Autodesk Inventor part; units mm, degrees
ref_plane "YZ Plane" through (0, 0, 0) normal (1, 0, 0) x (0, 1, 0)
ref_plane "XZ Plane" through (0, 0, 0) normal (0, 1, 0) x (-1, 0, 0)
ref_plane "XY Plane" through (0, 0, 0) normal (0, 0, 1) x (1, 0, 0)
sketch "Sketch1" plane through (0, 0, 0) normal (0, 0, 1) x (1, 0, 0)
  line L0 (0, 0) -> (13, 0)
  line L1 (13, 0) -> (13, 80)
  line L2 (13, 80) -> (0, 80)
  line L3 (0, 80) -> (0, 0)
  dimension "d0" = 80
  dimension "d1" = 13
extrude "Extrusion1" add sketch "Sketch1" along normal blind 58
sketch "Sketch2" plane through (0, 0, 58) normal (0, 0, 1) x (1, 0, 0)
  line L0 (10, 77) -> (3, 77)
  line L1 (3, 3) -> (10, 3)
  line L2 (10, 3) -> (10, 77)
  line L3 (13, 0) -> (13, 80)
  line L4 (13, 80) -> (0, 80)
  line L5 (0, 0) -> (13, 0)
  line L6 (0, 80) -> (0, 0)
  line L7 (0, 10) -> (3, 10)
  line L8 (3, 70) -> (0, 70)
  line L9 (0, 70) -> (0, 10)
  line L10 (3, 77) -> (3, 70)
  line L11 (3, 10) -> (3, 3)
  point P0 (0, 70)
  dimension "d4" = 3
  dimension "d5" = 3
  dimension "d6" = 3
  dimension "d8" = 10
  dimension "d9" = 10
extrude "Extrusion2" cut sketch "Sketch2" against normal through all contours L2 L1 L11 L7 L6 L8 L10 L0
sketch "Sketch3" plane through (13, 0, 0) normal (1, 0, 0) x (0, 0, -1)
  circle A0 centre (-40, 40) radius 4
  line L0 (-58, 0) -> (-58, 80)
  line L1 (0, 0) -> (-58, 0)
  line L2 (0, 0) -> (0, 80)
  dimension "d12" = 8
  dimension "d14" = 40
  dimension "d17" = 40
extrude "Extrusion3" cut sketch "Sketch3" against normal through all
properties part number "servo_mount" material "PC/ABS Plastic"
For this review, take the finished solid that the model builds, in its own axes (mm). A direction names the side the tool comes from. Round coordinates to 2 decimals unless told otherwise and drop trailing zeros. Order: outer loops, then holes, each group sorted by start corner. A loop starts at its lowest first (then second) coordinate and runs counter-clockwise, first axis right, second up.
Q1. We need section C-C, the plane x = 1.5. Give the boundary of the cut face in (y, z).
Findings below:
outline: (0, 0) - (10, 0) - (10, 58) - (0, 58) - close; (70, 0) - (80, 0) - (80, 58) - (70, 58) - close
Q2. Mouldability with a two-part tool opening along X and no side actions: class faces 4 (the flat face through (2, 70, 29)), 5 (the flat face through (3, 74, 29)), 6 (the flat face through (0, 75, 29)) as pulls with the +X half, pulls with the -X half, needs draft (parallel to the pull), parting line crosses it, or undercut.
Findings below:
face 4: needs draft
face 5: undercut
face 6: pulls with the -X half
Q3. We need section A-A, the plane y = 40. Give the boundary of the cut face in (x, z), plus the area to 3 significant figures.
Findings below:
outline: (10, 0) - (13, 0) - (13, 36) - (10, 36) - close; (10, 44) - (13, 44) - (13, 58) - (10, 58) - close
area: 150 mm2
Q4. Wall thickness on line 1 (Y direction, x = 1.5, z = 20); line 2 (Y direction, x = 11.7, z = 40); line 3 (X direction, y = 6.5, z = 17.5): over which ranges is each line inside the solid? List them lowest first.
Findings below:
line 1: y = 0 to 10, 70 to 80
line 2: y = 0 to 36, 44 to 80
line 3: x = 0 to 3, 10 to 13
Q5. We need section D-D, the plane z = 47.5. Give the boundary of the cut face in (x, y).
Findings below:
outline: (0, 0) - (13, 0) - (13, 80) - (0, 80) - (0, 70) - (3, 70) - (3, 77) - (10, 77) - (10, 3) - (3, 3) - (3, 10) - (0, 10) - close
Q6. Insertion check: P1, Ø10.5, axis at y = 40, z = 40, coming from the -X side. The pin has a flat end and moves straight along its axis. Give the tip position at first contact, or say it passes through.
Findings below:
P1: stops at x = 10
Q7. Machinability: for faces 1 (the flat face through (10.3, 40.2, 0)), 2 (the flat face through (1, 10, 29)), 3 (the flat face through (10, 39, 29)), which of the approach directions +Z, -Z, +X, -X, +Y, -Y give a long, thin tool a straight path to every point of the face, cutting with its end or side? Answer none if there is none.
Findings below:
face 1: -Z, +X, -X, +Y, -Y
face 2: +Z, -Z, -X
face 3: +Z, -Z
Q8. We need section B-B, the plane z = 40. Give the boundary of the cut face in (x, y), plus the area to 3 significant figures.
Findings below:
outline: (0, 0) - (13, 0) - (13, 36) - (10, 36) - (10, 3) - (3, 3) - (3, 10) - (0, 10) - close; (0, 70) - (3, 70) - (3, 77) - (10, 77) - (10, 44) - (13, 44) - (13, 80) - (0, 80) - close
area: 318 mm2
